from build123d import *

# Parameters (mm, degrees)
F1_DEPTH = 7.5
F2_R     = 0.99999


# Not quite as in the source:
# - a fillet or chamfer is up to 0.001 mm smaller than in the source, because OpenCascade refuses the exact size


with BuildPart() as f1:
    # F0 (on Front) → F1 (new body, symmetric)
    with BuildSketch(Plane.XZ):
        with BuildLine():
            Line((0, 25.4), (0, 3))
            ThreePointArc((0, 3), (0.8786796564, 0.8786796564), (3, 0))
            Line((3, 0), (25.4, 0))
            Line((25.4, 0), (25.4, 2))
            Line((25.4, 2), (3, 2))
            ThreePointArc((3, 2), (2.2928932188, 2.2928932188), (2, 3))
            Line((2, 3), (2, 25.4))
            Line((2, 25.4), (0, 25.4))
        make_face()
    extrude(amount=F1_DEPTH, both=True)

    # F2 (radius 1 in the source; OpenCascade refuses exactly that, so slightly less here)
    f2_edges = [f1.edges().sort_by_distance(p)[0] for p in [
        (2, 0, 25.4),
        (0, 0, 25.4),
    ]]
    fillet(f2_edges, radius=F2_R)


solid = f1.part
Here's how the part is built. I have some questions about the finished solid (model axes, mm). A direction names the side the tool comes from. Coordinates: 2 decimals unless noted, no trailing zeros. Order: outer loops, then holes, each group sorted by start corner. A loop starts at its lowest first (then second) coordinate and runs counter-clockwise, first axis right, second up.
Item 1: I need wall thicknesses on line 1 (X direction, y = 1.75, z = 5). Which ranges of the line are inside material? Lowest first, please.
Result sheet:
line 1: x = 0 to 2
Item 2: For faces 1 (the face through (14, 0, 2)), 2 (the face through (1, -7.5, 7)), which set-ups out of +Z, -Z, +X, -X, +Y, -Y let a thin tool reach every point of the face, with its end or its side?
Result sheet:
face 1: +Z, +X, +Y, -Y
face 2: +Z, -Z, +X, -X, -Y
Item 3: If we section it at B-B on z = 18.5: List the corners of the cut face in (x, y) for me, plus the area to 3 significant figures.
Result sheet:
outline: (0, -7.5) - (2, -7.5) - (2, 7.5) - (0, 7.5) - close
area: 30.0 mm2
Item 4: If we section it at C-C on x = 10: List the corners of the cut face in (y, z) for me.
Result sheet:
outline: (-7.5, 0) - (7.5, 0) - (7.5, 2) - (-7.5, 2) - close
Item 5: For P1, Ø3, axis at y = 1.5, z = 13, coming from the +X side; P2, Ø10, axis at x = 10, z = 15.5, coming from the -Y side; P3, Ø1.5, axis at x = 22.5, y = 1.5, coming from the -Z side; P4, Ø4, axis at x = 18, y = -6, coming from the +Z side, each with a flat end and sliding along its axis, tell me the tip position at first contact or that it passes through.
Result sheet:
P1: stops at x = 2
P2: passes through
P3: stops at z = 0
P4: stops at z = 2
